Could you check a few things on this model? Use its own coordinates, in mm. A direction names the side the tool comes from. Round coordinates to 2 decimals unless told otherwise and drop trailing zeros. Order: outer loops, then holes, each group sorted by start corner. A loop starts at its lowest first (then second) coordinate and runs counter-clockwise, first axis right, second up. Notation, with made-up numbers: (-14, 57.25) -> (27, 57.25) arc R22 cw to (27, 69.25) -> close; hole circle Ø2 at (47.5, 56.25). An arc over 180 degrees is marked (long way). Put each result on its own line as item: value. Start each with the question number.
from build123d import *

# Parameters (mm, degrees)
SKETCH1_W           = 250
SKETCH1_H           = 46
BOSS_EXTRUDE1_DEPTH = 6
SKETCH2_W           = 50
SKETCH2_H           = 6
CUT_EXTRUDE1_DEPTH  = 6
SKETCH3_R           = 13.5
CUT_EXTRUDE2_DEPTH  = 10


with BuildPart() as part:
    # Sketch1 → Boss-Extrude1 (new body)
    with BuildSketch(Plane.XY):
        Rectangle(SKETCH1_W, SKETCH1_H)
    extrude(amount=BOSS_EXTRUDE1_DEPTH)

    # Sketch2 → Cut-Extrude1 (cut)
    with BuildSketch(Plane.XY.offset(6)):
        with Locations((0, -20)):
            Rectangle(SKETCH2_W, SKETCH2_H)
        with Locations((-100, -20)):
            Rectangle(SKETCH2_W, SKETCH2_H)
        with Locations((100, -20)):
            Rectangle(SKETCH2_W, SKETCH2_H)
    extrude(amount=-CUT_EXTRUDE1_DEPTH, mode=Mode.SUBTRACT)

    # Sketch3 → Cut-Extrude2 (cut)
    with BuildSketch(Plane.XY.offset(6)):
        with Locations((-105, -1.5)):
            Circle(SKETCH3_R)
    extrude(amount=-CUT_EXTRUDE2_DEPTH, mode=Mode.SUBTRACT)


solid = part.part
1. I need wall thicknesses on L1, parallel to Y at x = -105, z = 2.45; L2, parallel to X at y = -0.5, z = 2.4; L3, parallel to X at y = -4.5, z = 0.95. Which ranges of each line are inside material? Lowest first, please.
2. Thinking about a two-plate mould opening in Y: for faces 5 (the face through (75, -20, 3)), 6 (the face through (-118.487, -0.906, 3.042)), 7 (the face through (50, -23, 3)), 8 (the face through (-2, 23, 3)), which applies, +Y half, -Y half, draft (parallel to the pull), parting line (faces both ways), or undercut?
3. For pin 1 Ø1.8 at (y, z) = (-21.5, 2) entering from -X; pin 2 Ø16 at (x, y) = (-105, -1.5) entering from +Z; pin 3 Ø1.8 at (x, z) = (-3, 3) entering from -Y, each with a flat end and sliding along its axis, tell me the tip position at first contact or that it passes through.
4. If we section it at B-B, the plane x = -105: Please give me the cut outline in (y, z).
5. If we section it at A-A, the plane y = -1.5: Please give me the cut outline in (x, z), then the cut area to 3 significant figures.
6. If we section it at C-C, the plane z = 1.85: Please give me the cut outline in (x, y).
7. Which directions (+Z, -Z, +X, -X, +Y, -Y) give clear straight access to the entire face, cutting with the end or side of a thin tool? Please do faces 1 (the face through (100, -17, 3)), 2 (the face through (-75, -20, 3)), 3 (the face through (-2, 0, 0)), 4 (the face through (-25, -20, 3)).
8. If we section it at D-D, the plane x = -21.5: Please give me the cut outline in (y, z), then the cut area to 3 significant figures.
Results below:
1. L1: -17 to -15, 12 to 23
1. L2: -125 to -118.46, -91.54 to 125
1. L3: -125 to -118.16, -91.84 to 125
2. face 5: draft
2. face 6: undercut
2. face 7: -Y half
2. face 8: +Y half
3. pin 1: x = -75
3. pin 2: through
3. pin 3: y = -17
4. outline: (-17, 0) -> (-15, 0) -> (-15, 6) -> (-17, 6) -> close; (12, 0) -> (23, 0) -> (23, 6) -> (12, 6) -> close
5. outline: (-125, 0) -> (-118.5, 0) -> (-118.5, 6) -> (-125, 6) -> close; (-91.5, 0) -> (125, 0) -> (125, 6) -> (-91.5, 6) -> close
5. area: 1,340 mm2
6. outline: (-125, -17) -> (-75, -17) -> (-75, -23) -> (-25, -23) -> (-25, -17) -> (25, -17) -> (25, -23) -> (75, -23) -> (75, -17) -> (125, -17) -> (125, 23) -> (-125, 23) -> close; hole circle Ø27 at (-105, -1.5)
7. face 1: +Z, -Z, +X, -Y
7. face 2: +Z, -Z, -X, -Y
7. face 3: -Z, +X, -X, +Y, -Y
7. face 4: +Z, -Z, -Y
8. outline: (-17, 0) -> (23, 0) -> (23, 6) -> (-17, 6) -> close
8. area: 240 mm2
